The listing builds one solid part. Answer for the finished solid, in the listing's coordinates (mm). Face numbers are marked on the shaded views. A direction names the side the tool comes from. Round coordinates to 2 decimals unless told otherwise and drop trailing zeros. Write each loop counter-clockwise with the first axis right and the second up, starting at its lowest first coordinate (ties: lowest second). Pieces come first, ordered by that corner, then holes.
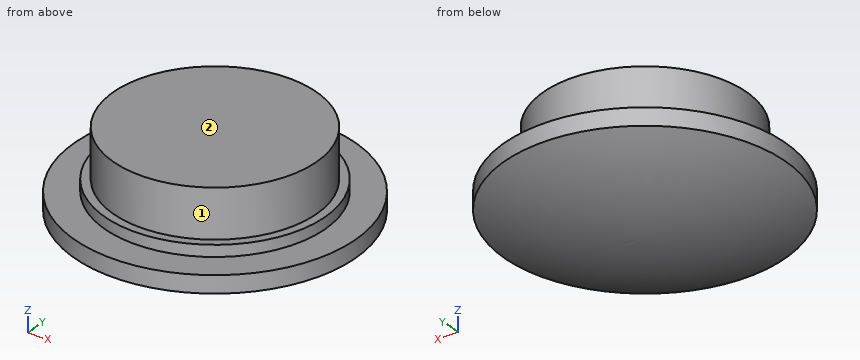
from build123d import *

# Parameters (mm, degrees)
SKETCH6_R          = 6.864817117
CUT_EXTRUDE2_DEPTH = 3.3
SKETCH5_R          = 15.702559167
CUT_EXTRUDE3_DEPTH = 40


# Read off the part's stored shape, not the designer's step: Split1
with BuildPart() as part:
    # Sketch1 → Revolve2 (revolve)
    with BuildSketch(Plane(origin=(0, 0, 0), x_dir=(0, 0, -1), z_dir=(1, 0, 0)), mode=Mode.PRIVATE) as revolve2_sk:
        with BuildLine():
            Line((1.771e-06, 9.5), (1.771e-06, 7.445611339))
            Line((1.771e-06, 7.445611339), (-0.771464581, 7.445611339))
            Line((-0.771464581, 7.445611339), (-0.771464581, 6.864817117))
            Line((-0.771464581, 6.864817117), (-4.066354879, 6.864817117))
            Line((-4.066354879, 6.864817117), (-4.066354879, 8.484339467))
            Line((-4.066354879, 8.484339467), (-4.975618005, 9.546154997))
            Line((-4.975618005, 9.546154997), (-7.06424338, 9.546154997))
            Line((-7.06424338, 9.546154997), (-7.767897919, 10.954193429))
            Line((-7.767897919, 10.954193429), (-9.164037876, 10.954193429))
            Line((-9.164037876, 10.954193429), (-9.945876251, 9.546154997))
            Line((-9.945876251, 9.546154997), (-9.945876251, 8))
            Line((-9.945876251, 8), (-19.896053439, 8))
            Line((-19.896053439, 8), (-20.566354879, 7.426001631))
            Line((-20.566354879, 7.426001631), (-23.121440557, 7.426001631))
            Line((-23.121440557, 7.426001631), (-23.682625072, 6.864817117))
            Line((-23.682625072, 6.864817117), (-23.682625072, 6.383537324))
            Line((-23.682625072, 6.383537324), (-27.0133813, 6.383537324))
            Line((-27.0133813, 6.383537324), (-27.0133813, 5.464238658))
            Line((-27.0133813, 5.464238658), (-31.931960755, 5.464238658))
            Line((-31.931960755, 5.464238658), (-31.931960755, 1.447456583))
            Line((-31.931960755, 1.447456583), (-38.111348046, 1.447456583))
            Line((-38.111348046, 1.447456583), (-38.931960755, 1.037362766))
            Line((-38.931960755, 1.037362766), (-38.931960755, 0))
            Line((-38.931960755, 0), (2.933645121, 0))
            ThreePointArc((2.933645121, 0), (2.489100327, 4.831124101), (1.170397182, 9.5))
            Line((1.170397182, 9.5), (1.771e-06, 9.5))
        make_face()
    revolve(revolve2_sk.sketch.rotate(Axis((0, 0, 38.931960755), (0, 0, -1)), 90), axis=Axis((0, 0, 38.931960755), (0, 0, -1)))


with BuildPart() as body_2:
    # Split1: the piece on the far side of the plane
    add(part.part)
    split(bisect_by=Plane.XY.offset(4.066354879), keep=Keep.BOTTOM)


with BuildPart() as part_1:
    add(part.part)

    # Split1
    split(bisect_by=Plane.XY.offset(4.066354879), keep=Keep.TOP)

    # Sketch6 → Cut-Extrude2 (cut)
    with BuildSketch(Plane(origin=(0, 0, 4.066354879), x_dir=(-1, 0, 0), z_dir=(0, 0, -1))):
        with Locations(Location((0, 0, 0), (0, 0, 180))):
            Circle(SKETCH6_R)
    extrude(amount=-CUT_EXTRUDE2_DEPTH, mode=Mode.SUBTRACT)

    # Sketch5 → Cut-Extrude3 (cut)
    with BuildSketch(Plane(origin=(0, 0, 4.066354879), x_dir=(-1, 0, 0), z_dir=(0, 0, -1))):
        Circle(SKETCH5_R)
    extrude(amount=-CUT_EXTRUDE3_DEPTH, mode=Mode.SUBTRACT)


solid = body_2.part
1. A tool of negligible diameter and unlimited length cuts with its end or side. For the marked faces 1 and 2, from which of +Z, -Z, +X, -X, +Y, -Y can it reach the whole face along a straight path? Write none if from no direction.
Geometry says:
face 1: +Z
face 2: +Z, +X, -X, +Y, -Y
2. Section A-A on z = -0.5 is taken. Determine the outline of the cut face in (x, y).
Geometry says:
outline: circle Ø19 at (0, 0)
3. Straight lines are drawn through the part: line 1 along Y through (x, z) = (0, -1); line 2 along X through (y, z) = (-6, -0.75); line 3 along Z through (x, y) = (3, 6.5). For each, find the intervals that lie inside material, in ascending order.
Geometry says:
line 1: y = -9.5 to 9.5
line 2: x = -7.37 to 7.37
line 3: z = -1.95 to 0.77
4. Section B-B on z = 2 is taken. Determine the outline of the cut face in (x, y).
Geometry says:
outline: circle Ø13.73 at (0, 0)
5. Given pin 1 (1 mm diameter, centred on x = 4.5, y = 7, fed in from -Z); pin 2 (8 mm diameter, centred on x = 0.5, y = -4.5, fed in from -Z); pin 3 (1.5 mm diameter, centred on x = 3, z = -1, fed in from +Y), each flat-ended and moving along its own axis, determine where each tip first touches the part or whether it passes through.
Geometry says:
pin 1: stops at z = -1.75
pin 2: stops at z = -2.93
pin 3: stops at y = 9.23
